Model file for the job. Use its own axes, mm. A direction names the side the tool comes from. Coordinates: 2 decimals unless noted, no trailing zeros. Write each loop counter-clockwise with the first axis right and the second up, starting at its lowest first coordinate (ties: lowest second). Pieces come first, ordered by that corner, then holes. Notation, with made-up numbers: (-25, 47.5) -> (-13, 47.5) arc R21 ccw to (-13, 86.5) -> close; hole circle Ø3 at (54, 58.25). An arc over 180 degrees is marked (long way). Answer as a JSON object with one key per item and string values. Group by question number.
from build123d import *

# Parameters (mm, degrees)
SKETCH1_W            = 14.224
SKETCH1_H            = 9.3472
BOSS_EXTRUDE1_DEPTH  = 10.922
SKETCH2_W            = 11.43
SKETCH2_H            = 8.458212498
BOSS_EXTRUDE2_DEPTH  = 3.048
SKETCH3_W            = 2.25993982
SKETCH3_H            = 1.702901352
SKETCH3_W_2          = 2.231792691
SKETCH3_H_2          = 1.576239268
BOSS_EXTRUDE3_DEPTH  = 1.524
SKETCH4_R            = 0.254
BOSS_EXTRUDE4_DEPTH  = 6.604
LPATTERN1_COUNT      = 3
LPATTERN1_PITCH      = 2.54
LPATTERN1_COUNT_DIR2 = 2
LPATTERN1_PITCH_DIR2 = 4.8514
SKETCH5_W            = 10.16
SKETCH5_H            = 1.778
CUT_EXTRUDE1_DEPTH   = 7.493
CHAMFER1_SIZE        = 1.524
FILLET1_R            = 1.524


with BuildPart() as part:
    # Sketch1 → Boss-Extrude1 (new body)
    with BuildSketch(Plane(origin=(0, 0, 0), x_dir=(1, 0, 0), z_dir=(0, 1, 0))):
        Rectangle(SKETCH1_W, SKETCH1_H)
    extrude(amount=-BOSS_EXTRUDE1_DEPTH)

    # Sketch2 → Boss-Extrude2 (add)
    with BuildSketch(Plane.XZ.offset(10.922)):
        Rectangle(SKETCH2_W, SKETCH2_H)
    extrude(amount=BOSS_EXTRUDE2_DEPTH)

    # Sketch3 → Boss-Extrude3 (add)
    with BuildSketch(Plane.XZ.offset(13.97)):
        with Locations((-4.58503009, 3.377655573)):
            Rectangle(SKETCH3_W, SKETCH3_H)
        with Locations((4.599103655, 3.377655573)):
            Rectangle(SKETCH3_W_2, SKETCH3_H)
        with Locations((4.599103655, -3.440986615)):
            Rectangle(SKETCH3_W_2, SKETCH3_H_2)
        with Locations((-4.58503009, -3.440986615)):
            Rectangle(SKETCH3_W, SKETCH3_H_2)
    extrude(amount=BOSS_EXTRUDE3_DEPTH)

    # Sketch4 → Boss-Extrude4 (add)
    with BuildSketch(Plane.XZ.offset(13.97)):
        with Locations((-2.54, -2.4257)):
            Circle(SKETCH4_R)
    boss_extrude4 = extrude(amount=BOSS_EXTRUDE4_DEPTH)

    # LPattern1: Boss-Extrude4 3 × 2
    with Locations(*[(i * LPATTERN1_PITCH, 0, j * LPATTERN1_PITCH_DIR2) for i in range(LPATTERN1_COUNT) for j in range(LPATTERN1_COUNT_DIR2) if (i, j) != (0, 0)]):
        add(boss_extrude4)

    # Sketch5 → Cut-Extrude1 (cut)
    with BuildSketch(Plane(origin=(0, 0, 0), x_dir=(1, 0, 0), z_dir=(0, 1, 0))):
        Rectangle(SKETCH5_W, SKETCH5_H)
    extrude(amount=-CUT_EXTRUDE1_DEPTH, mode=Mode.SUBTRACT)

    # Chamfer1
    chamfer1_edges = [part.edges().sort_by_distance(p)[0] for p in [
        (-5.08, 0, 0),
        (5.08, 0, 0),
    ]]
    chamfer(chamfer1_edges, length=CHAMFER1_SIZE)

    # Fillet1
    fillet1_edges = [part.edges().sort_by_distance(p)[0] for p in [
        (0, 0, 0.889),
        (0, 0, -0.889),
    ]]
    fillet(fillet1_edges, radius=FILLET1_R)


solid = part.part
(1) Cut at C-C on z = 3. List the corners of the cut face in (x, y) (3 decimals), plus the area to 3 significant figures.
(2) 3-axis set-ups, long thin cutter, end or side, ignore diameter. For faces 1 (the face through (5, -15, -2.653)), 2 (the face through (3.483, -15, 3)), 3 (the face through (-5, -15, 2.526)), 4 (the face through (-0.09, -0.43, 1.35)), 5 (the face through (0, -13, 4.229)): which of +Z, -Z, +X, -X, +Y, -Y reach the whole face in a straight line?
(3) Cut at A-A on y = -6.75. List the corners of the cut face in (x, z), plus the area to 3 significant figures.
(4) Wall check: probe 1 along X at (y, z) = (-5, -0.5); probe 2 along Z at (x, y) = (-5, -2); probe 3 along Y at (x, z) = (4.5, 3). Give the ranges that are in metal, low to high.
(5) Cut at D-D on y = -17. List the corners of the cut face in (x, z).
(6) Cut at B-B on x = 4.25. List the corners of the cut face in (y, z).
(7) Pull direction X, two halves, no side cores. Call faces 6 (the face through (-5, -15.494, 3)), 7 (the face through (-5.08, -4, 0)), 8 (the face through (7.112, -5, 0)): released by +X, released by -X, zero draft, split by the parting line, or undercut.
(8) Pin check, flat tips, straight feed: pin 1 (1.7 mm diameter, centred on x = -4.5, y = -14.5, fed in from -Z); pin 2 (0.8 mm diameter, centred on y = -15, z = -3.5, fed in from +X) (3 decimals); pin 3 (0.9 mm diameter, centred on x = -4, z = 3.5, fed in from -Y). Stop position of each tip, or through.
Results found:
{
 "1": {"outline": "(-7.112, -10.922) -> (-5.715, -10.922) -> (-5.715, -15.494) -> (-3.455, -15.494) -> (-3.455, -13.97) -> (3.483, -13.97) -> (3.483, -15.494) -> (5.715, -15.494) -> (5.715, -10.922) -> (7.112, -10.922) -> (7.112, 0) -> (-7.112, 0) -> close", "area": "197 mm²"},
 "2": {"face 1": "+X, -Y", "face 2": "+Z, -Z, -Y", "face 3": "-X, -Y", "face 4": "+Y", "face 5": "+Z, +X, -X, -Y"},
 "3": {"outline": "(-7.11, -4.67) -> (7.11, -4.67) -> (7.11, 4.67) -> (-7.11, 4.67) -> close; hole (-5.08, -0.89) -> (5.08, -0.89) -> (5.08, 0.89) -> (-5.08, 0.89) -> close", "area": "115 mm²"},
 "4": {"probe 1": "x = -7.11 to -5.08, 5.08 to 7.11", "probe 2": "z = -4.67 to -0.89, 0.89 to 4.67", "probe 3": "y = -15.49 to 0"},
 "5": {"outline": "circle Ø0.51 at (-2.54, -2.43); circle Ø0.51 at (-2.54, 2.43); circle Ø0.51 at (0, -2.43); circle Ø0.51 at (0, 2.43); circle Ø0.51 at (2.54, -2.43); circle Ø0.51 at (2.54, 2.43)"},
 "6": {"outline": "(-15.49, -4.23) -> (-10.92, -4.23) -> (-10.92, -4.67) -> (0, -4.67) -> (0, -2.41) arc R1.52 ccw to (-1.52, -0.89) -> (-7.49, -0.89) -> (-7.49, 0.89) -> (-1.52, 0.89) arc R1.52 ccw to (0, 2.41) -> (0, 4.67) -> (-10.92, 4.67) -> (-10.92, 4.23) -> (-15.49, 4.23) -> (-15.49, 2.53) -> (-13.97, 2.53) -> (-13.97, -2.65) -> (-15.49, -2.65) -> close"},
 "7": {"face 6": "zero draft", "face 7": "undercut", "face 8": "released by +X"},
 "8": {"pin 1": "stops at z = -4.23", "pin 2": "stops at x = 5.715", "pin 3": "stops at y = -15.49"}
}
